from build123d import *

# Parameters (mm, degrees)
SKETCH1_W           = 36.5125
SKETCH1_H           = 4.7625
BOSS_EXTRUDE1_DEPTH = 25.4
SKETCH2_W           = 12.7
SKETCH2_H           = 1.5875
CUT_EXTRUDE1_DEPTH  = 25.4
SKETCH3_W           = 16.8275
SKETCH3_H           = 25.4
BOSS_EXTRUDE2_DEPTH = 0.79375
SKETCH4_W           = 36.5125
SKETCH4_H           = 25.4
BOSS_EXTRUDE3_DEPTH = 0.79375


with BuildPart() as part:
    # Sketch1 → Boss-Extrude1 (new body)
    with BuildSketch(Plane(origin=(0, 0, 0), x_dir=(1, 0, 0), z_dir=(0, 1, 0))):
        Rectangle(SKETCH1_W, SKETCH1_H)
    extrude(amount=BOSS_EXTRUDE1_DEPTH)

    # Sketch2 → Cut-Extrude1 (cut)
    with BuildSketch(Plane(origin=(0, 25.4, 0), x_dir=(1, 0, 0), z_dir=(0, 1, 0))):
        with Locations((0, -1.5875)):
            Rectangle(SKETCH2_W, SKETCH2_H)
    extrude(amount=-CUT_EXTRUDE1_DEPTH, mode=Mode.SUBTRACT)

    # Sketch3 → Boss-Extrude2 (add)
    with BuildSketch(Plane(origin=(0, 0, -2.38125), x_dir=(-1, 0, 0), z_dir=(0, 0, -1))):
        with Locations((0, 12.7)):
            Rectangle(SKETCH3_W, SKETCH3_H)
    extrude(amount=BOSS_EXTRUDE2_DEPTH)

    # Sketch4 → Boss-Extrude3 (add)
    with BuildSketch(Plane(origin=(0, 0, -3.175), x_dir=(-1, 0, 0), z_dir=(0, 0, -1))):
        with Locations((0, 12.7)):
            Rectangle(SKETCH4_W, SKETCH4_H)
    extrude(amount=BOSS_EXTRUDE3_DEPTH)


solid = part.part
Here's how the part is built. I have some questions about the finished solid (model axes, mm). A direction names the side the tool comes from. Round coordinates to 2 decimals unless told otherwise and drop trailing zeros. Order: outer loops, then holes, each group sorted by start corner. A loop starts at its lowest first (then second) coordinate and runs counter-clockwise, first axis right, second up. Notation, with made-up numbers: M 20,1.5 L 38,1.5 A27 ccw 38,36.5 Z; hole C 18,85.25 d9. An arc over 180 degrees is marked long. Return JSON: item names as keys, results as strings. Group by question number.
1. If we section it at B-B on z = 1.25: List the corners of the cut face in (x, y) for me.
2. Please list where these lines run through material, in increasing order: probe 1 along Z at (x, y) = (-15, 7) (3 decimals); probe 2 along X at (y, z) = (13.5, 1.75); probe 3 along X at (y, z) = (6.25, -2.75).
3. On a 3-axis mill with a long thin cutter (end or side, diameter ignored), from which of +Z, -Z, +X, -X, +Y, -Y can I reach the whole of each face in a straight line? I mean faces 5 (the face through (0, 25.4, -1)), 6 (the face through (-6.35, 13, 2)), 7 (the face through (13, 13, -3.175)). Say none if no direction works.
4. If we section it at C-C on y = 13.75: List the corners of the cut face in (x, z) for me (3 decimals).
5. If we section it at D-D on x = 1: List the corners of the cut face in (y, z) for me.
6. If we section it at A-A on x = -14: List the corners of the cut face in (y, z) for me (3 decimals), then the cut area to 3 significant figures.
7. I'm going to push a flat-ended pin straight in: pin 1 Ø6.5 at (x, y) = (-1, 18.5) entering from +Z. Where does the tip first touch, or does it pass through?
8. If we mould it in two halves opening along Z, with no side actions, what happens to faces 1 (the face through (-13, 13, -3.175)), 2 (the face through (-13, 13, -2.381)), 3 (the face through (0, 0, -1)), 4 (the face through (0, 13, -3.969))? For each: pulls with the +Z half, pulls with the -Z half, needs draft (parallel to the pull), parting line crosses it, or undercut.
Reply:
{
 "1": {"outline": "M -18.26,0 L -6.35,0 L -6.35,25.4 L -18.26,25.4 Z; M 6.35,0 L 18.26,0 L 18.26,25.4 L 6.35,25.4 Z"},
 "2": {"probe 1": "-3.969 to -3.175, -2.381 to 2.381", "probe 2": "-18.26 to -6.35, 6.35 to 18.26", "probe 3": "-8.41 to 8.41"},
 "3": {"face 5": "+Z, -Z, +X, -X, +Y", "face 6": "+Z, +Y, -Y", "face 7": "+X, +Y, -Y"},
 "4": {"outline": "M -18.256,-3.969 L 18.256,-3.969 L 18.256,-3.175 L 8.414,-3.175 L 8.414,-2.381 L 18.256,-2.381 L 18.256,2.381 L 6.35,2.381 L 6.35,0.794 L -6.35,0.794 L -6.35,2.381 L -18.256,2.381 L -18.256,-2.381 L -8.414,-2.381 L -8.414,-3.175 L -18.256,-3.175 Z"},
 "5": {"outline": "M 0,-3.97 L 25.4,-3.97 L 25.4,0.79 L 0,0.79 Z"},
 "6": {"outline": "M 0,-3.969 L 25.4,-3.969 L 25.4,-3.175 L 0,-3.175 Z; M 0,-2.381 L 25.4,-2.381 L 25.4,2.381 L 0,2.381 Z", "area": "141 mm^2"},
 "7": {"pin 1": "z = 0.79"},
 "8": {"face 1": "undercut", "face 2": "undercut", "face 3": "needs draft", "face 4": "pulls with the -Z half"}
}
